Geometry: final body of the model. Coordinates: model frame, mm. Give positions to 0.01 mm unless a question says otherwise; leave off trailing zeros. Write each loop counter-clockwise with the first axis right and the second up, starting at its lowest first coordinate (ties: lowest second). Pieces come first, ordered by that corner, then holes.
Q1. Cut plane B-B on y = 55. Return the cut outline in (x, z), plus the area to 3 significant figures.
Q2. Pin query (flat end, axial travel): pin 1 (8 mm diameter, centred on y = 18.5, z = 2, fed in from -X); pin 2 (1.9 mm diameter, centred on y = 67, z = 4.5, fed in from -X); pin 3 (4 mm diameter, centred on y = 79, z = 3, fed in from -X). Return the tip coordinate at first contact, or that it passes through.
Q3. Line query: L1, parallel to Y at x = 32, z = 13.75; L2, parallel to Z at x = 66, y = 7; L3, parallel to Y at x = 95.5, z = 13. Output: solid intervals per line, ascending.
Q4. Cut plane A-A on x = 24. Return the cut outline in (y, z).
Q5. Cut plane C-C on x = 188.5. Return the cut outline in (y, z).
```python
from build123d import *

# Parameters (mm, degrees)
BOSS_EXTRUDE1_DEPTH = 15.24
BOSS_EXTRUDE2_DEPTH = 6.35
SKETCH3_W           = 76.2
SKETCH3_H           = 12.7
BOSS_EXTRUDE3_DEPTH = 7.62
CUT_EXTRUDE1_DEPTH  = 76.2
CUT_EXTRUDE2_DEPTH  = 280.00035691
FILLET1_R           = 1.27
FILLET2_R           = 5.08
SKETCH6_W           = 228.6
SKETCH6_H           = 2.54
BOSS_EXTRUDE4_DEPTH = 7.62


with BuildPart() as part:
    # Sketch1 → Boss-Extrude1 (new body)
    with BuildSketch(Plane.XY):
        Polygon((0, 0), (228.6, 0), (228.6, 7.366), (0, 7.366), (0, 4.826), (76.2, 4.826), (76.2, 2.54), (0, 2.54), align=None)
    extrude(amount=BOSS_EXTRUDE1_DEPTH)

    # Sketch2 → Boss-Extrude2 (add)
    with BuildSketch(Plane.XY):
        Polygon((228.6, 7.366), (228.6, 159.766), (82.55, 7.366), (89.586126025, 7.366), (223.52, 147.123085887), (223.52, 7.366), align=None)
    extrude(amount=BOSS_EXTRUDE2_DEPTH)

    # Sketch3 → Boss-Extrude3 (add)
    with BuildSketch(Plane.XY):
        with Locations((38.1, 6.35)):
            Rectangle(SKETCH3_W, SKETCH3_H)
    extrude(amount=BOSS_EXTRUDE3_DEPTH)

    # Sketch5 → Cut-Extrude1 (cut)
    with BuildSketch(Plane.ZY):
        Polygon((7.62, 2.54), (2.54, 2.54), (2.54, 12.7), (5.08, 12.7), (5.08, 4.826), (7.62, 4.826), align=None)
    extrude(amount=-CUT_EXTRUDE1_DEPTH, mode=Mode.SUBTRACT)

    # Sketch7 → Cut-Extrude2 (cut, through all)
    with BuildSketch(Plane.XY.offset(7.62)):
        Polygon((76.2, 7.366), (66.961240992, 12.7), (76.2, 12.7), align=None)
    extrude(amount=-CUT_EXTRUDE2_DEPTH, mode=Mode.SUBTRACT)

    # Fillet1
    fillet1_edges = [part.edges().sort_by_distance(p)[0] for p in [
        (38.1, 4.826, 5.08),
        (38.1, 2.54, 2.54),
    ]]
    fillet(fillet1_edges, radius=FILLET1_R)

    # Fillet2
    fillet2_edges = [part.edges().sort_by_distance(p)[0] for p in [
        (223.52, 7.366, 3.175),
        (82.55, 7.366, 3.175),
        (223.52, 147.123085887, 3.175),
    ]]
    fillet(fillet2_edges, radius=FILLET2_R)

    # Sketch6 → Boss-Extrude4 (add)
    with BuildSketch(Plane(origin=(0, 7.366, 0), x_dir=(1, 0, 0), z_dir=(0, 1, 0))):
        with Locations((114.3, -13.97)):
            Rectangle(SKETCH6_W, SKETCH6_H)
    extrude(amount=BOSS_EXTRUDE4_DEPTH)


solid = part.part
```
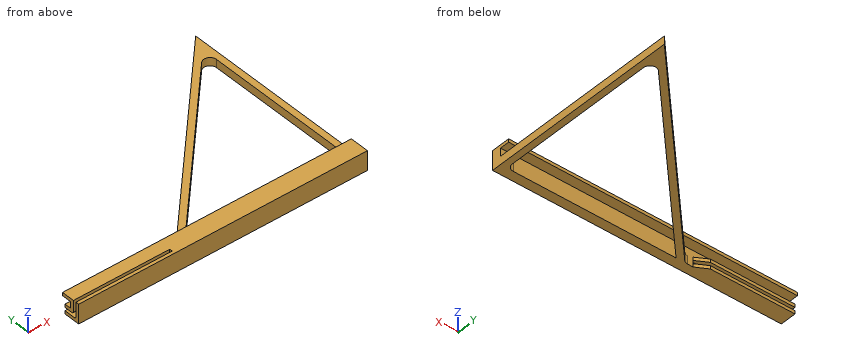
Data:
1. outline: (128.2, 0) - (135.24, 0) - (135.24, 6.35) - (128.2, 6.35) - close; (223.52, 0) - (228.6, 0) - (228.6, 6.35) - (223.52, 6.35) - close
1. area: 76.9 mm2
2. pin 1: stops at x = 89.39
2. pin 2: stops at x = 138.79
2. pin 3: stops at x = 149.28
3. L1: y = 0 to 2.54, 4.83 to 14.99
3. L2: z = 0 to 2.54, 5.08 to 15.24
3. L3: y = 0 to 14.99
4. outline: (0, 0) - (12.7, 0) - (12.7, 2.54) - (3.81, 2.54) arc R1.27 cw to (2.54, 3.81) - (2.54, 15.24) - (0, 15.24) - close; (4.83, 6.35) arc R1.27 ccw to (6.1, 5.08) - (12.7, 5.08) - (12.7, 7.62) - (7.37, 7.62) - (7.37, 12.7) - (14.99, 12.7) - (14.99, 15.24) - (4.83, 15.24) - close
5. outline: (0, 0) - (7.37, 0) - (7.37, 12.7) - (14.99, 12.7) - (14.99, 15.24) - (0, 15.24) - close; (110.58, 0) - (117.92, 0) - (117.92, 6.35) - (110.58, 6.35) - close
